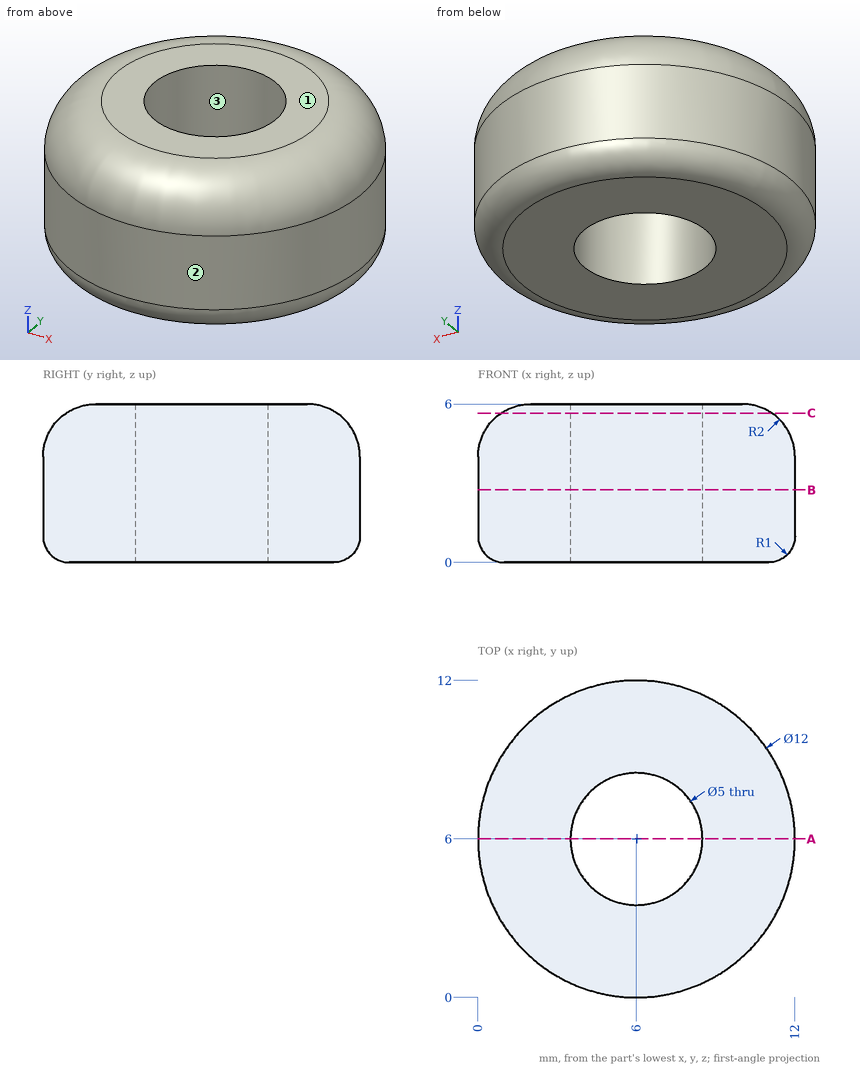
Print and shaded views of the part. All mm, measured from the part's lowest x, y and z. Coordinates: 2 decimals unless noted, no trailing zeros. Order: outer loops, then holes, each group sorted by start corner. A loop starts at its lowest first (then second) coordinate and runs counter-clockwise, first axis right, second up.
Item 1: Saw through at B-B on z = 2.75. List the corners of the cut face in (x, y).
Filled in:
outline: circle Ø12 at (6, 6); hole circle Ø5 at (6, 6)
Item 2: Drop flat-ended pins along their axis: pin 1 Ø1 at (y, z) = (9, 3.5) entering from +X; pin 2 Ø1 at (x, z) = (5, 2) entering from +Y; pin 3 Ø1.5 at (x, z) = (4, 0.5) entering from -Y. Give the stop position or say it passes through.
Filled in:
pin 1: stops at x = 11.45
pin 2: stops at y = 11.98
pin 3: stops at y = 0.16
Item 3: Saw through at A-A on y = 6. List the corners of the cut face in (x, z).
Filled in:
outline: (0, 1) arc R1 ccw to (1, 0) - (3.5, 0) - (3.5, 6) - (2, 6) arc R2 ccw to (0, 4) - close; (8.5, 0) - (11, 0) arc R1 ccw to (12, 1) - (12, 4) arc R2 ccw to (10, 6) - (8.5, 6) - close
Item 4: Saw through at C-C on z = 5.65. List the corners of the cut face in (x, y).
Filled in:
outline: circle Ø10.26 at (6, 6); hole circle Ø5 at (6, 6)
Item 5: Drill centre lines: L1, parallel to Y at x = 6, z = 2.4; L2, parallel to Y at x = 6.5, z = 1.4; L3, parallel to X at y = 7, z = 2.8. Where is each one in solid material? Low to high.
Filled in:
L1: y = 0 to 3.5, 8.5 to 12
L2: y = 0.02 to 3.55, 8.45 to 11.98
L3: x = 0.08 to 3.71, 8.29 to 11.92
Item 6: Mould opens along X. For the marked faces 1, 2 and 3 say: released by +X, released by -X, zero draft, split by the parting line, or undercut.
Filled in:
face 1: zero draft
face 2: split by the parting line
face 3: undercut
